Geometry: final body of the model. Coordinates: model frame, mm. Round coordinates to 2 decimals unless told otherwise and drop trailing zeros. Loops run counter-clockwise (first coordinate to the right, second up) from the corner with the lowest first, then second, coordinate; pieces in that order, holes last. Notation, with made-up numbers: M 60,-22 L 97,-22 A5 cw 97,-14 Z; hole C 44.5,75 d9. An arc over 180 degrees is marked long. Answer as a JSON object with one key per item and string values.
```python
from build123d import *

# Parameters (mm, degrees)
SKETCH1_R           = 2.38125
BOSS_EXTRUDE1_DEPTH = 3.175
SKETCH2_R           = 2.38125
CUT_EXTRUDE1_DEPTH  = 3.175


with BuildPart() as part:
    # Sketch1 → Boss-Extrude1 (new body)
    with BuildSketch(Plane.XY):
        with BuildLine():
            Line((-6.35, 0), (-6.35, 30.1625))
            ThreePointArc((-6.35, 30.1625), (0, 36.5125), (6.35, 30.1625))
            Line((6.35, 30.1625), (6.35, 0))
            ThreePointArc((6.35, 0), (0, -6.35), (-6.35, 0))
        make_face()
        Circle(SKETCH1_R, mode=Mode.SUBTRACT)
        with Locations((0, 30.1625)):
            Circle(SKETCH1_R, mode=Mode.SUBTRACT)
    extrude(amount=BOSS_EXTRUDE1_DEPTH)

    # Sketch2 → Cut-Extrude1 (cut)
    with BuildSketch(Plane.XY.offset(3.175)):
        with Locations((0, 15.08125)):
            Circle(SKETCH2_R)
    extrude(amount=-CUT_EXTRUDE1_DEPTH, mode=Mode.SUBTRACT)


solid = part.part
```
1) Line query: probe 1 along Y at (x, z) = (0, 1.85); probe 2 along Y at (x, z) = (0.5, 1.65); probe 3 along X at (y, z) = (31.5, 0.75). Output: solid intervals per line, ascending.
Geometry results:
{"probe 1": "-6.35 to -2.38, 2.38 to 12.7, 17.46 to 27.78, 32.54 to 36.51", "probe 2": "-6.33 to -2.33, 2.33 to 12.75, 17.41 to 27.83, 32.49 to 36.49", "probe 3": "-6.21 to -1.97, 1.97 to 6.21"}
2) Cut plane C-C on z = 2.05. Return the cut outline in (x, y), and give its area (3 significant figures).
Geometry results:
{"outline": "M -6.35,0 A6.35 ccw 6.35,0 L 6.35,30.16 A6.35 ccw -6.35,30.16 Z; hole C 0,0 d4.76; hole C 0,15.08 d4.76; hole C 0,30.16 d4.76", "area": "456 mm2"}
3) Cut plane B-B on y = 15.5. Return the cut outline in (x, z) (3 decimals), and give its area (3 significant figures).
Geometry results:
{"outline": "M -6.35,0 L -2.344,0 L -2.344,3.175 L -6.35,3.175 Z; M 2.344,0 L 6.35,0 L 6.35,3.175 L 2.344,3.175 Z", "area": "25.4 mm2"}
4) First-contact query: pin 1 (4.5 mm diameter, centred on x = 0, y = 0, fed in from +Z). Flat tip, straight axial feed; report the tip coordinate or a pass-through.
Geometry results:
{"pin 1": "through"}
5) Cut plane D-D on x = 4.5. Return the cut outline in (y, z) (3 decimals).
Geometry results:
{"outline": "M -4.48,0 L 34.643,0 L 34.643,3.175 L -4.48,3.175 Z"}
6) Cut plane A-A on x = 0. Count the separate pieces of the cut face and the enclosed holes in it, and give its area (3 significant figures).
Geometry results:
{"separate pieces": "4", "enclosed holes": "0", "area": "90.7 mm2"}
7) Pull-direction query (X, two-part tool) for faces 1 (the face through (-3, 15, 0)), 2 (the face through (0.14, -6.35, 1.57)), 3 (the face through (-1.89, -1.45, 1.57)), 4 (the face through (-0.31, 17.442, 1.61)); classes: +X half, -X half, draft (parallel to the pull), parting line (faces both ways), or undercut.
Geometry results:
{"face 1": "draft", "face 2": "parting line", "face 3": "undercut", "face 4": "undercut"}
